```python
from build123d import *

# Parameters (mm, degrees)
EXTRUDE_1_DEPTH           = 27
CUT_EXTRUDE_1_DEPTH       = 27
SKETCH_3_R                = 2.5000000000000013
EXTRUDE_2_DEPTH           = 2
CUT_EXTRUDE_START         = -2
SKETCH_4_R                = 8.5
SKETCH_4_R_2              = 2.5000000000000018
CUT_EXTRUDE_2_DEPTH       = 2
SKETCH_5_R                = 8.5
CUT_EXTRUDE_3_DEPTH       = 17
SKETCH_9_W                = 19
SKETCH_9_H                = 0.7371254741666728
CUT_EXTRUDE_7_DEPTH       = 4
CUT_EXTRUDE_8_DEPTH       = 0.906172
EXTRUDE_START             = 2
SKETCH_13_R               = 2.5000000000000004
EXTRUDE_4_DEPTH           = 2
SKETCH_14_W               = 3
SKETCH_14_H               = 7.375961595364039
SKETCH_14_W_2             = 2.9999999999999964
CUT_EXTRUDE_10_DEPTH      = 30
CUT_EXTRUDE_11_DEPTH      = 37.95471984311929
CUT_EXTRUDE_11_DEPTH_BACK = 37.95471984311929
FILLET_3_R                = 6
SKETCH_19_W               = 2.3759615953640427
SKETCH_19_H               = 13
CUT_EXTRUDE_13_DEPTH      = 37.95471984311929
SKETCH_18_R               = 7.499999999999999
EXTRUDE_5_DEPTH           = 2
EXTRUDE_START_2           = -2
SKETCH_20_R               = 7.499999999999999
EXTRUDE_6_DEPTH           = 2
SKETCH_21_W               = 27.916060476025446
SKETCH_21_H               = 6.853449812850004
CUT_EXTRUDE_14_DEPTH      = 44.16278511667507
CUT_EXTRUDE_15_DEPTH      = 41.84856377041868
CUT_EXTRUDE_15_DEPTH_BACK = 41.84856377041868
SKETCH_22_R               = 2.5999999999999996
FILLET_4_R                = 0.6
FILLET_5_R                = 0.6
FILLET_6_R                = 1
FILLET_7_R                = 0.5
SKETCH_23_R               = 2.5000000000000004
CUT_EXTRUDE_16_DEPTH      = 0.75
CUT_EXTRUDE_START_2       = -0.75
SKETCH_25_R               = 2.5000000000000013
CUT_EXTRUDE_17_DEPTH      = 0.75
FILLET_8_R                = 0.5
SKETCH_27_W               = 15
SKETCH_27_H               = 4.175939890720404
CUT_EXTRUDE_18_DEPTH      = 4
EXTRUDE_8_DEPTH           = 5
FILLET_9_R                = 1
SKETCH_29_W               = 2.9999999999999964
SKETCH_29_H               = 12.999999999999996
SKETCH_29_W_2             = 3
EXTRUDE_9_DEPTH           = 0.5
CHAMFER_1_SIZE            = 2


with BuildPart() as part:
    # 草圖1 → 填料-伸長1 (new body)
    with BuildSketch(Plane.XY):
        Polygon((-1.8124414345344562, 12.355214230576285), (23.187558565465547, 12.355214230576285), (23.187558565465547, -0.6447857694237141), (-1.8124414345344548, -0.6447857694237142), align=None)
        Polygon((3.1875585654655443, 9.355214230576284), (18.187558565465544, 9.355214230576284), (18.187558565465544, 1.355214230576286), (3.187558565465545, 1.355214230576286), align=None, mode=Mode.SUBTRACT)
    extrude(amount=EXTRUDE_1_DEPTH)

    # 草圖2 → 除料-伸長1 (cut)
    with BuildSketch(Plane(origin=(0, 12.355214230576285, 0), x_dir=(1, 0, 0), z_dir=(0, 1, 0))):
        Polygon((1.1875585654655443, 0), (20.187558565465547, 0), (20.187558565465547, -8), (1.1875585654655452, -8), align=None)
    extrude(amount=-CUT_EXTRUDE_1_DEPTH, mode=Mode.SUBTRACT)

    # 草圖3 → 填料-伸長2 (add)
    with BuildSketch(Plane.ZY.offset(-20.187558565465547)):
        with Locations(Location((4.5, 6.855214230576285, 0), (0, 0, 180))):
            Circle(SKETCH_3_R)
    extrude(amount=EXTRUDE_2_DEPTH)

    # 草圖4 → 除料-伸長2 (cut)
    with BuildSketch(Plane.ZY.offset(-18.187558565465547).offset(CUT_EXTRUDE_START)):
        with Locations((4.500000000000004, 6.855214230576285)):
            Circle(SKETCH_4_R)
        with Locations(Location((4.500000000000004, 6.855214230576285, 0), (0, 0, 180))):
            Circle(SKETCH_4_R_2, mode=Mode.SUBTRACT)
    extrude(amount=CUT_EXTRUDE_2_DEPTH, mode=Mode.SUBTRACT)

    # 草圖5 → 除料-伸長3 (cut)
    with BuildSketch(Plane.ZY.offset(-18.187558565465547)):
        with Locations((4.500000000000004, 6.855214230576285)):
            Circle(SKETCH_5_R)
    extrude(amount=CUT_EXTRUDE_3_DEPTH, mode=Mode.SUBTRACT)

    # 草圖9 → 除料-伸長7 (cut)
    with BuildSketch(Plane(origin=(0, 12.355214230576285, 0), x_dir=(1, 0, 0), z_dir=(0, 1, 0))):
        with Locations((10.687558565465551, -11.349303435491194)):
            Rectangle(SKETCH_9_W, SKETCH_9_H)
    extrude(amount=-CUT_EXTRUDE_7_DEPTH, mode=Mode.SUBTRACT)

    # 草圖10 → 除料-伸長8 (cut)
    with BuildSketch(Plane(origin=(0, 0, 11.717866172574531), x_dir=(-1, 0, 0), z_dir=(0, 0, -1))):
        Polygon((-20.18755856546555, 12.355214230576285), (-1.1875585654655494, 12.355214230576285), (-1.1875585654655487, 9.355214230576284), (-20.18755856546555, 9.355214230576284), align=None)
    extrude(amount=-CUT_EXTRUDE_8_DEPTH, mode=Mode.SUBTRACT)

    # 草圖13 → 填料-伸長4 (add)
    with BuildSketch(Plane(origin=(1.1875585654655443, 0, -1.3e-16), x_dir=(-1.1e-16, 0, -1), z_dir=(1, 0, -1.1e-16)).offset(EXTRUDE_START)):
        with Locations((-4.5, 6.855214230576285)):
            Circle(SKETCH_13_R)
    extrude(amount=-EXTRUDE_4_DEPTH)

    # 草圖14 → 除料-伸長10 (cut)
    with BuildSketch(Plane(origin=(0, 12.355214230576285, 0), x_dir=(1, 0, 0), z_dir=(0, 1, 0))):
        with Locations((-0.31244143453445605, -23.312019202317984)):
            Rectangle(SKETCH_14_W, SKETCH_14_H)
        with Locations((21.687558565465544, -23.312019202317984)):
            Rectangle(SKETCH_14_W_2, SKETCH_14_H)
        Polygon((3.1875585654655425, -27), (18.187558565465547, -27), (18.187558565465547, -19.624038404635964), (3.1875585654655443, -19.624038404635964), align=None)
    extrude(amount=-CUT_EXTRUDE_10_DEPTH, mode=Mode.SUBTRACT)

    # 草圖15 → 除料-伸長11 (cut, two sides: drawn at the far end of the back side and taken through both)
    with BuildSketch(Plane.ZY.offset(-20.187558565465547).offset(-CUT_EXTRUDE_11_DEPTH_BACK)):
        Polygon((0, 9.00201797372982), (3.3531962568464273, 12.355214230576285), (0, 12.355214230576285), align=None)
    extrude(amount=CUT_EXTRUDE_11_DEPTH + CUT_EXTRUDE_11_DEPTH_BACK, mode=Mode.SUBTRACT)

    # 圓角3
    fillet_3_edges = [part.edges().sort_by_distance(p)[0] for p in [
        (-0.31244143453445616, 9.00201797372982, 0),
        (21.687558565465547, 9.00201797372982, 0),
    ]]
    fillet(fillet_3_edges, radius=FILLET_3_R)

    # 草圖19 → 除料-伸長13 (cut, through all)
    with BuildSketch(Plane.ZY.offset(-1.187558565465544)):
        with Locations((25.812019202317984, 5.855214230576285)):
            Rectangle(SKETCH_19_W, SKETCH_19_H)
    extrude(amount=-CUT_EXTRUDE_13_DEPTH, mode=Mode.SUBTRACT)

    # 草圖18 → 填料-伸長5 (add)
    with BuildSketch(Plane(origin=(20.187558565465547, 0, 0), x_dir=(0, 0, -1), z_dir=(1, 0, 0))):
        with Locations((-24.624038404635964, 6.855214230576285)):
            Circle(SKETCH_18_R)
    extrude(amount=-EXTRUDE_5_DEPTH)

    # 草圖20 → 填料-伸長6 (add)
    with BuildSketch(Plane.ZY.offset(-1.187558565465544).offset(EXTRUDE_START_2)):
        with Locations((24.624038404635964, 6.855214230576285)):
            Circle(SKETCH_20_R)
    extrude(amount=EXTRUDE_6_DEPTH)

    # 草圖21 → 除料-伸長14 (cut, through all)
    with BuildSketch(Plane(origin=(23.187558565465547, 0, 0), x_dir=(0, 0, -1), z_dir=(1, 0, 0))):
        with Locations((-28.1917606773101, 15.781939137001288)):
            Rectangle(SKETCH_21_W, SKETCH_21_H)
    extrude(amount=-CUT_EXTRUDE_14_DEPTH, mode=Mode.SUBTRACT)

    # 草圖22 → 除料-伸長15 (cut, two sides: drawn at the far end of the back side and taken through both)
    with BuildSketch(Plane(origin=(20.187558565465547, 0, 0), x_dir=(0, 0, -1), z_dir=(1, 0, 0)).offset(-CUT_EXTRUDE_15_DEPTH_BACK)):
        with Locations((-24.624038404635964, 6.8552142305762835)):
            Circle(SKETCH_22_R)
    extrude(amount=CUT_EXTRUDE_15_DEPTH + CUT_EXTRUDE_15_DEPTH_BACK, mode=Mode.SUBTRACT)

    # 圓角4
    fillet_4_edges = [part.edges().sort_by_distance(p)[0] for p in [
        (20.187558565465547, 6.855214230576285, 27.224038404635962),
    ]]
    fillet(fillet_4_edges, radius=FILLET_4_R)

    # 圓角5
    fillet_5_edges = [part.edges().sort_by_distance(p)[0] for p in [
        (1.1875585654655438, 6.855214230576285, 27.224038404635962),
    ]]
    fillet(fillet_5_edges, radius=FILLET_5_R)

    # 圓角6
    # the kernel refuses this fillet: 1 mm, written as the material it adds along each edge
    with BuildSketch(Plane(origin=(18.187558565465544, 9.355214230576284, 19.624038404635964), x_dir=(3.55e-15, -1, 1.066e-14), z_dir=(5.1e-16, -1.066e-14, -1))) as fillet_6_piece_1_section:
        with BuildLine():
            CenterArc((FILLET_6_R, FILLET_6_R), FILLET_6_R, 180, 90.00000000000023)
            Line((-3.55e-15, FILLET_6_R), (0, 0))
            Line((0, 0), (FILLET_6_R, 0))
        make_face()
    fillet_6_piece_1 = extrude(amount=9.499999999999957, mode=Mode.PRIVATE)
    fillet_6_piece_1 = split(fillet_6_piece_1, bisect_by=Plane(origin=(17.960107802534193, 9.130564344096692, 12.624038172574531), z_dir=(0, 0, 1)), keep=Keep.TOP, mode=Mode.PRIVATE)
    fillet_6_piece_1 = fillet_6_piece_1 - Plane(origin=(17.96010780253419, 6.855214230576285, 4.5), x_dir=(2.4e-16, 0, 1), z_dir=(1, 0, -2.4e-16)) * Cylinder(8.5, 23, mode=Mode.PRIVATE)
    add(fillet_6_piece_1)
    with BuildSketch(Plane(origin=(3.187558565465544, 9.355214230576284, 10.124038404635964), x_dir=(0, -1, 0), z_dir=(0, 0, 1))) as fillet_6_piece_2_section:
        with BuildLine():
            CenterArc((FILLET_6_R, FILLET_6_R), FILLET_6_R, 180, 90)
            Line((0, FILLET_6_R), (0, 0))
            Line((0, 0), (FILLET_6_R, 0))
        make_face()
    fillet_6_piece_2 = extrude(amount=9.5, mode=Mode.PRIVATE)
    fillet_6_piece_2 = split(fillet_6_piece_2, bisect_by=Plane(origin=(3.4150094343401456, 9.130564406809754, 12.624038172574531), z_dir=(0, 0, 1)), keep=Keep.TOP, mode=Mode.PRIVATE)
    fillet_6_piece_2 = fillet_6_piece_2 - Plane(origin=(3.415009434340142, 6.855214230576285, 4.5000000000000036), x_dir=(2.4e-16, 0, 1), z_dir=(1, 0, -2.4e-16)) * Cylinder(8.5, 23, mode=Mode.PRIVATE)
    add(fillet_6_piece_2)

    # 圓角7
    fillet_7_edges = [part.edges().sort_by_distance(p)[0] for p in [
        (10.687558565465999, 9.355214230576284, 19.624038404635964),
        (3.4804517842794525, 9.062321011762547, 19.624038404636),
        (17.894665346652545, 9.062321011762547, 19.624038404636),
    ]]
    fillet(fillet_7_edges, radius=FILLET_7_R)

    # 草圖23 → 除料-伸長16 (cut)
    with BuildSketch(Plane(origin=(3.1875585654655443, 0, -3.5e-16), x_dir=(-1.1e-16, 0, -1), z_dir=(1, 0, -1.1e-16))):
        with Locations(Location((-4.5, 6.855214230576285, 0), (0, 0, 180))):
            Circle(SKETCH_23_R)
    extrude(amount=-CUT_EXTRUDE_16_DEPTH, mode=Mode.SUBTRACT)

    # 草圖25 → 除料-伸長17 (cut)
    with BuildSketch(Plane.ZY.offset(-18.187558565465547).offset(CUT_EXTRUDE_START_2)):
        with Locations(Location((4.500000000000004, 6.855214230576285, 0), (0, 0, 180))):
            Circle(SKETCH_25_R)
    extrude(amount=CUT_EXTRUDE_17_DEPTH, mode=Mode.SUBTRACT)

    # 圓角8
    fillet_8_edges = [part.edges().sort_by_distance(p)[0] for p in [
        (2.437558565465545, 6.855214230576286, 7),
        (18.937558565465547, 6.855214230576284, 7.000000000000001),
    ]]
    fillet(fillet_8_edges, radius=FILLET_8_R)

    # 草圖27 → 除料-伸長18 (cut)
    with BuildSketch(Plane.XY.offset(19.624038404635964)):
        with Locations((10.687558565465544, 10.267244285216083)):
            Rectangle(SKETCH_27_W, SKETCH_27_H)
    extrude(amount=-CUT_EXTRUDE_18_DEPTH, mode=Mode.SUBTRACT)

    # 草圖28 → 填料-伸長8 (add)
    with BuildSketch(Plane.XY.offset(19.624038404635964)):
        Polygon((18.187558565465547, -0.6447857694237141), (3.1875585654655443, -0.6447857694237141), (3.1875585654655434, 1.355214230576286), (18.187558565465547, 1.3552142305762875), align=None)
    extrude(amount=EXTRUDE_8_DEPTH)

    # 圓角9
    fillet_9_edges = [part.edges().sort_by_distance(p)[0] for p in [
        (18.187558565465544, 1.3552142305762809, 17.8023895515219),
        (3.1875585654655443, 1.355214230576286, 17.802389551521912),
    ]]
    fillet(fillet_9_edges, radius=FILLET_9_R)

    # 草圖29 → 填料-伸長9 (add)
    with BuildSketch(Plane.XY.offset(19.624038404635964)):
        with Locations((21.687558565465544, 5.8552142305762835)):
            Rectangle(SKETCH_29_W, SKETCH_29_H)
        with Locations((-0.31244143453445605, 5.8552142305762835)):
            Rectangle(SKETCH_29_W_2, SKETCH_29_H)
    extrude(amount=EXTRUDE_9_DEPTH)

    # 導角1
    chamfer_1_edges = [part.edges().sort_by_distance(p)[0] for p in [
        (21.687558565465547, -0.6447857694237141, 0),
        (21.687558565465547, -0.6447857694237141, 20.124038404635964),
        (-0.31244143453445616, -0.6447857694237141, 20.124038404635964),
        (-0.31244143453445616, -0.6447857694237142, 0),
    ]]
    chamfer(chamfer_1_edges, length=CHAMFER_1_SIZE)


solid = part.part
```
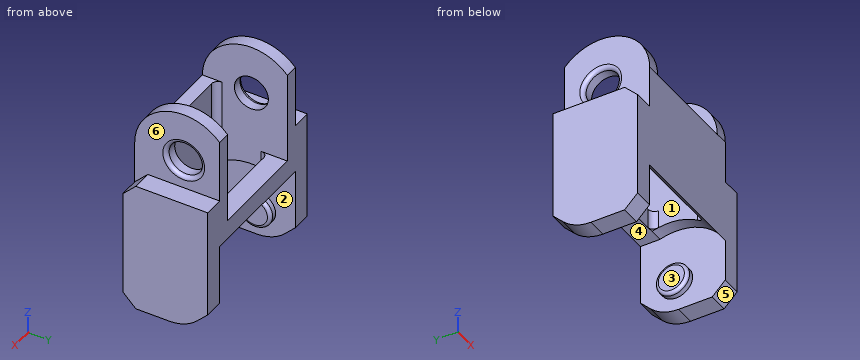
Input: part model. Units: mm. Frame: model coordinates. Face numbers are marked on the shaded views. A direction names the side the tool comes from. Coordinates: 2 decimals unless noted, no trailing zeros. Loops run counter-clockwise (first coordinate to the right, second up) from the corner with the lowest first, then second, coordinate; pieces in that order, holes last. Notation, with made-up numbers: M 84.5,36.25 L 140.5,36.25 A15 cw 140.5,54.25 Z; hole C 89,-36.75 d2. An arc over 180 degrees is marked long. One line per item, written item: value.
(1) Reachability of the marked faces 1, 2 and 3 from +Z, -Z, +X, -X, +Y, -Y: full face, straight path, thin tool, end or side. Return the list, or none.
Filled in:
face 1: +Z
face 2: none
face 3: -Z, +Y, -Y
(2) Line query: line 1 along Y through (x, z) = (15.75, 14); line 2 along X through (y, z) = (3.5, 7); line 3 along X through (y, z) = (9, 28). Output: solid intervals per line, ascending. Write a range as from..to.
Filled in:
line 1: -0.64..1.36, 9.36..12.36
line 2: -1.81..1.19, 20.19..23.19
line 3: 1.19..3.19, 18.19..20.19
(3) Pull-direction query (X, two-part tool) for the marked faces 4, 5 and 6; classes: +X half, -X half, draft (parallel to the pull), parting line (faces both ways), or undercut.
Filled in:
face 4: undercut
face 5: draft
face 6: +X half
(4) Section D-D (z = 18.5). Output: boundary loops of the cut face in (x, y).
Filled in:
outline: M -1.81,-0.27 L 1.19,-0.27 L 1.19,-0.64 L 20.19,-0.64 L 20.19,-0.27 L 23.19,-0.27 L 23.19,12.36 L 18.19,12.36 L 18.19,2.36 A1 cw 17.19,1.36 L 4.19,1.36 A1 cw 3.19,2.36 L 3.19,12.36 L -1.81,12.36 Z
(5) Section C-C (y = 0.75). Output: boundary loops of the cut face in (x, z).
Filled in:
outline: M -1.81,0.61 L 1.19,0.61 L 1.19,10.41 L 20.19,10.41 L 20.19,0.61 L 23.19,0.61 L 23.19,19.52 L 20.19,19.52 L 20.19,28.98 L 18.19,28.98 L 18.19,24.62 L 3.19,24.62 L 3.19,28.98 L 1.19,28.98 L 1.19,19.52 L -1.81,19.52 Z
(6) Section B-B (x = 14.25). Output: boundary loops of the cut face in (y, z), and give its area (3 significant figures).
Filled in:
outline: M -0.64,8.5 A8.5 cw 1.36,10.98 L 1.36,24.62 L -0.64,24.62 Z; M 9.36,12.62 L 12.36,12.62 L 12.36,15.62 L 9.36,15.62 Z
area: 38.4 mm^2
(7) Pin query (flat end, axial travel): pin 1 (0.9 mm diameter, centred on x = -0.5, y = 5.5, fed in from +Z); pin 2 (1.5 mm diameter, centred on x = 7.5, y = 10, fed in from -Z); pin 3 (1.5 mm diameter, centred on x = 9.5, y = 1.5, fed in from +Z). Return the tip coordinate at first contact, or that it passes through.
Filled in:
pin 1: z = 20.12
pin 2: z = 12.62
pin 3: z = 24.62
(8) Section A-A (z = 4.5). Output: boundary loops of the cut face in (x, y).
Filled in:
outline: M -1.81,-0.64 L 1.19,-0.64 L 1.19,4.36 L 1.94,4.36 A0.5 ccw 2.44,4.86 L 2.44,8.86 A0.5 ccw 1.94,9.36 L 1.19,9.36 L 1.19,12.36 L -1.81,12.36 Z; M 18.94,4.86 A0.5 ccw 19.44,4.36 L 20.19,4.36 L 20.19,-0.64 L 23.19,-0.64 L 23.19,12.36 L 20.19,12.36 L 20.19,9.36 L 19.44,9.36 A0.5 ccw 18.94,8.86 Z
